```python
from build123d import *

# Parameters (mm, degrees)
F0_W     = 11.6
F0_H     = 50
F1_DEPTH = 2.4
F2_R     = 2.5
F2_W     = 0.5
F2_H     = 40
F3_DEPTH = 25
F4_R     = 1


with BuildPart() as f1:
    # F0 (on Top) → F1 (new body)
    with BuildSketch(Plane.XY):
        Rectangle(F0_W, F0_H)
    extrude(amount=F1_DEPTH)

    # F2 (on face) → F3 (cut)
    with BuildSketch(Plane.XY.offset(2.4)):
        with Locations((5.8, 20)):
            Circle(F2_R)
        with Locations((5.55, -5)):
            Rectangle(F2_W, F2_H)
        with Locations((-5.8, 20)):
            Circle(F2_R)
        with Locations((-5.55, -5)):
            Rectangle(F2_W, F2_H)
    extrude(amount=-F3_DEPTH, mode=Mode.SUBTRACT)

    # F4
    f4_edges = [f1.edges().sort_by_distance(p)[0] for p in [
        (5.8, 22.5, 1.2),
        (5.8, 17.5, 1.2),
        (-5.8, 22.5, 1.2),
        (-5.8, 17.5, 1.2),
        (5.8, 25, 1.2),
        (-5.8, 25, 1.2),
    ]]
    fillet(f4_edges, radius=F4_R)


solid = f1.part
```
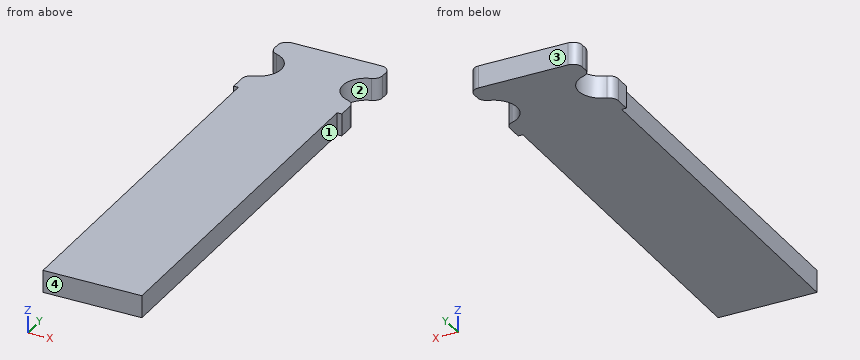
CAD build for the part. Positions are in the model's coordinates, mm. Face numbers are marked on the shaded views. Round coordinates to 2 decimals unless told otherwise and drop trailing zeros. Loops run counter-clockwise (first coordinate to the right, second up) from the corner with the lowest first, then second, coordinate; pieces in that order, holes last. Notation, with made-up numbers: M 46,49 L 54,49 A8 ccw 54,54 Z; hole C -38.5,-5.75 d4. An arc over 180 degrees is marked long. Return JSON: item names as keys, results as strings. Group by question number.
(1) Saw through at A-A, the plane x = -4. List the corners of the cut face in (y, z), and give its area (3 significant figures).
(2) Wall check: probe 1 along X at (y, z) = (4, 1.85); probe 2 along Y at (x, z) = (4.25, 0.45); probe 3 along Y at (x, z) = (-5, 0.3). Give the ranges that are in metal, low to high. Write a range as [from, to].
(3) Drop a flat-ended pin along its axis: P1, Ø0.7, axis at y = -4, z = 1.5, coming from the -X side. Give the stop position or say it passes through.
(4) Mould opens along Y. For the marked faces 1, 2, 3 and 4 say: +Y half, -Y half, draft (parallel to the pull), parting line (faces both ways), or undercut.
(5) Saw through at D-D, the plane y = 19. List the corners of the cut face in (x, z), and give its area (3 significant figures).
(6) Saw through at B-B, the plane z = 2. List the corners of the cut face in (x, y), and give its area (3 significant figures).
(7) Saw through at C-C, the plane y = -4.5. List the corners of the cut face in (x, z).
Answer list:
{
 "1": {"outline": "M -25,0 L 18.27,0 L 18.27,2.4 L -25,2.4 Z; M 21.73,0 L 25,0 L 25,2.4 L 21.73,2.4 Z", "area": "112 mm2"},
 "2": {"probe 1": "[-5.3, 5.3]", "probe 2": "[-25, 18.04], [21.96, 25]", "probe 3": "[-25, 17.63], [22.37, 24.98]"},
 "3": {"P1": "x = -5.3"},
 "4": {"face 1": "draft", "face 2": "undercut", "face 3": "+Y half", "face 4": "-Y half"},
 "5": {"outline": "M -3.51,0 L 3.51,0 L 3.51,2.4 L -3.51,2.4 Z", "area": "16.8 mm2"},
 "6": {"outline": "M -5.8,15 L -5.3,15 L -5.3,-25 L 5.3,-25 L 5.3,15 L 5.8,15 L 5.8,16.65 A1 ccw 5.09,17.6 A2.5 cw 5.09,22.4 A1 ccw 5.8,23.35 L 5.8,24 A1 ccw 4.8,25 L -4.8,25 A1 ccw -5.8,24 L -5.8,23.35 A1 ccw -5.09,22.4 A2.5 cw -5.09,17.6 A1 ccw -5.8,16.65 Z", "area": "519 mm2"},
 "7": {"outline": "M -5.3,0 L 5.3,0 L 5.3,2.4 L -5.3,2.4 Z"}
}
